CAD build for the part. Positions are in the model's coordinates, mm. Coordinates: 2 decimals unless noted, no trailing zeros. Loops run counter-clockwise (first coordinate to the right, second up) from the corner with the lowest first, then second, coordinate; pieces in that order, holes last. Notation, with made-up numbers: M 33.5,-33 L 48.5,-33 A20 cw 48.5,-25 Z; hole C -10,16 d6. An arc over 180 degrees is marked long. Answer as a JSON object with one key per item and string values. Group by question number.
```python
from build123d import *

# Parameters (mm, degrees)
SKETCH1_W            = 95
SKETCH1_H            = 71
BOSS_EXTRUDE1_DEPTH  = 4
SKETCH2_R            = 3
BOSS_EXTRUDE2_DEPTH  = 7.5
SKETCH3_R            = 1.775
CUT_EXTRUDE1_DEPTH   = 64.736204248
SKETCH4_R            = 1.05
CUT_EXTRUDE2_DEPTH   = 64.13718185
LPATTERN1_COUNT      = 9
LPATTERN1_PITCH      = 4
LPATTERN1_COUNT_DIR2 = 9
LPATTERN1_PITCH_DIR2 = 4


with BuildPart() as part:
    # Sketch1 → Boss-Extrude1 (new body)
    with BuildSketch(Plane(origin=(0, 0, 0), x_dir=(1, 0, 0), z_dir=(0, 1, 0))):
        with Locations((4.168563349, 0.002299833)):
            Rectangle(SKETCH1_W, SKETCH1_H)
    extrude(amount=BOSS_EXTRUDE1_DEPTH)

    # Sketch2 → Boss-Extrude2 (add)
    with BuildSketch(Plane(origin=(0, 4, 0), x_dir=(1, 0, 0), z_dir=(0, 1, 0))):
        with Locations(Location((-38.831436651, -30.997700167, 0), (0, 0, 90))):
            Circle(SKETCH2_R)
        with Locations(Location((-38.831436651, 31.002299833, 0), (0, 0, 90))):
            Circle(SKETCH2_R)
        with Locations(Location((47.168563349, 31.002299833, 0), (0, 0, 90))):
            Circle(SKETCH2_R)
        with Locations(Location((47.168563349, -30.997700167, 0), (0, 0, 90))):
            Circle(SKETCH2_R)
    extrude(amount=BOSS_EXTRUDE2_DEPTH)

    # Sketch3 → Cut-Extrude1 (cut, through all)
    with BuildSketch(Plane(origin=(0, 11.5, 0), x_dir=(1, 0, 0), z_dir=(0, 1, 0))):
        with Locations(Location((-38.831436651, 31.002299833, 0), (0, 0, 270))):
            Circle(SKETCH3_R)
        with Locations(Location((-38.831436651, -30.997700167, 0), (0, 0, 270))):
            Circle(SKETCH3_R)
        with Locations(Location((47.168563349, -30.997700167, 0), (0, 0, 270))):
            Circle(SKETCH3_R)
        with Locations(Location((47.168563349, 31.002299833, 0), (0, 0, 270))):
            Circle(SKETCH3_R)
    extrude(amount=-CUT_EXTRUDE1_DEPTH, mode=Mode.SUBTRACT)

    # Sketch4 → Cut-Extrude2 (cut, through all)
    with BuildSketch(Plane(origin=(0, 4, 0), x_dir=(1, 0, 0), z_dir=(0, 1, 0))):
        with Locations(Location((-25.831436651, 23.502299833, 0), (0, 0, 270))):
            Circle(SKETCH4_R)
    cut_extrude2 = extrude(amount=-CUT_EXTRUDE2_DEPTH, mode=Mode.SUBTRACT)

    # LPattern1: Cut-Extrude2 9 × 9
    with Locations(*[(i * LPATTERN1_PITCH, 0, j * LPATTERN1_PITCH_DIR2) for i in range(LPATTERN1_COUNT) for j in range(LPATTERN1_COUNT_DIR2) if (i, j) != (0, 0)]):
        add(cut_extrude2, mode=Mode.SUBTRACT)


solid = part.part
```
Item 1: Pull direction X, two halves, no side cores. Call faces 1 (the flat face through (51.669, 2, 0)), 2 (the cylindrical face through (-22.856, 2.028, 4.27)), 3 (the flat face through (-43.331, 2, 0)): released by +X, released by -X, zero draft, split by the parting line, or undercut.
Item 2: Pin check, flat tips, straight feed: pin 1 (12 mm diameter, centred on x = 14.5, z = -21.5, fed in from +Y); pin 2 (4 mm diameter, centred on x = 38.5, y = 6.5, fed in from -Z). Stop position of each tip, or through.
Item 3: Drill centre line: L1, parallel to Y at x = 21, z = 7.5. Where is it in solid material? Low to high. Write a range as from..to.
Item 4: Slice it at B-B, the plane z = -23.5. Count the separate pieces of the cut face and the enclosed holes in it, then the cut area to 3 significant figures.
Item 5: Slice it at A-A, the plane y = 9.25. Write the cut outline in (x, z) (3 decimals).
Item 6: Slice it at D-D, the plane z = 18.5. Write the cut outline in (x, y).
Item 7: Slice it at C-C, the plane x = 10.5. Write the cut outline in (y, z), then the cut area to 3 significant figures.
Computed:
{
 "1": {"face 1": "released by +X", "face 2": "undercut", "face 3": "released by -X"},
 "2": {"pin 1": "y = 4", "pin 2": "through"},
 "3": {"L1": "0..4"},
 "4": {"separate pieces": "10", "enclosed holes": "0", "area": "304 mm2"},
 "5": {"outline": "C -38.831,-31.002 d6; C -38.831,30.998 d6; C 47.169,-31.002 d6; C 47.169,30.998 d6; hole C -38.831,-31.002 d3.55; hole C -38.831,30.998 d3.55; hole C 47.169,-31.002 d3.55; hole C 47.169,30.998 d3.55"},
 "6": {"outline": "M -43.33,0 L 51.67,0 L 51.67,4 L -43.33,4 Z"},
 "7": {"outline": "M 0,-35.5 L 4,-35.5 L 4,35.5 L 0,35.5 Z", "area": "284 mm2"}
}
